Read the model definition and answer for the solid it produces. Units are mm, in the model's axes. A direction names the side the tool comes from. Give positions to 0.01 mm unless a question says otherwise; leave off trailing zeros. Write each loop counter-clockwise with the first axis right and the second up, starting at its lowest first coordinate (ties: lowest second). Pieces come first, ordered by that corner, then holes.
```python
from build123d import *

# Parameters (mm, degrees)
SKETCH1_W                      = 55.88
SKETCH1_H                      = 12.7
BOSS_EXTRUDE1_DEPTH            = 3.81
SKETCH2_W                      = 9.525
SKETCH2_H                      = 12.7
BOSS_EXTRUDE2_DEPTH            = 16.51
F_8_0_199_DIAMETER_HOLE1_D     = 5.0546
F_8_0_199_DIAMETER_HOLE1_DEPTH = 7.112
F_8_0_199_DIAMETER_HOLE1_TIP   = 1.518555042


with BuildPart() as part:
    # Sketch1 → Boss-Extrude1 (new body)
    with BuildSketch(Plane(origin=(0, 0, 0), x_dir=(1, 0, 0), z_dir=(0, 1, 0))):
        with Locations((-27.94, 6.35)):
            Rectangle(SKETCH1_W, SKETCH1_H)
    extrude(amount=BOSS_EXTRUDE1_DEPTH)

    # Sketch2 → Boss-Extrude2 (add)
    with BuildSketch(Plane(origin=(0, 3.81, 0), x_dir=(1, 0, 0), z_dir=(0, 1, 0))):
        with Locations((-51.1175, 6.35)):
            Rectangle(SKETCH2_W, SKETCH2_H)
        with Locations((-4.7625, 6.35)):
            Rectangle(SKETCH2_W, SKETCH2_H)
    extrude(amount=BOSS_EXTRUDE2_DEPTH)

    # #8 (0.199) Diameter Hole1
    with Locations(Plane(origin=(0, 20.32, 0), x_dir=(1, 0, 0), z_dir=(0, 1, 0))):
        with Locations((-50.8254, 6.505248616), (-5.0546, 6.505248616)):
            Hole(F_8_0_199_DIAMETER_HOLE1_D / 2, depth=F_8_0_199_DIAMETER_HOLE1_DEPTH)
            with Locations((0, 0, -(F_8_0_199_DIAMETER_HOLE1_DEPTH + F_8_0_199_DIAMETER_HOLE1_TIP / 2))):  # 118° drill point
                Cone(0, F_8_0_199_DIAMETER_HOLE1_D / 2, F_8_0_199_DIAMETER_HOLE1_TIP, mode=Mode.SUBTRACT)


solid = part.part
```
Item 1: Section C-C (z = -2.5) is taken. Write down the section's boundary in (x, y) (3 decimals), and give its area (3 significant figures).
Result set:
outline: (-55.88, 0) - (0, 0) - (0, 20.32) - (-9.525, 20.32) - (-9.525, 3.81) - (-46.355, 3.81) - (-46.355, 20.32) - (-55.88, 20.32) - close
area: 527 mm2
Item 2: Section A-A (y = 7) is taken. Write down the section's boundary in (x, z) (3 decimals).
Result set:
outline: (-55.88, -12.7) - (-46.355, -12.7) - (-46.355, 0) - (-55.88, 0) - close; (-9.525, -12.7) - (0, -12.7) - (0, 0) - (-9.525, 0) - close
Item 3: Which of the six approach directions +Z, -Z, +X, -X, +Y, -Y give full straight-line access (tool end or side, diameter ignored) to faces 1 (the flat face through (-53.3, 20.32, -5)), 2 (the cylindrical face through (-4.73, 16.71, -9.01)), 3 (the flat face through (-46.355, 12, -6))?
Result set:
face 1: +Z, -Z, +X, -X, +Y
face 2: +Y
face 3: +Z, -Z, +Y
Item 4: Section D-D (x = -11.5) is taken. Write down the section's boundary in (y, z).
Result set:
outline: (0, -12.7) - (3.81, -12.7) - (3.81, 0) - (0, 0) - close
Item 5: Determine the mould class of faces 4 (the flat face through (-55.88, 10, -6)), 5 (the flat face through (-2.7, 20.32, -5)), 6 (the flat face through (-9.525, 12, -6)), 7 (the conical face through (-4.819, 11.953, -6.875)) for opening direction X: pulls with the +X half, pulls with the -X half, needs draft (parallel to the pull), parting line crosses it, or undercut.
Result set:
face 4: pulls with the -X half
face 5: needs draft
face 6: undercut
face 7: undercut
Item 6: Section B-B (y = 16.25) is taken. Write down the section's boundary in (x, z) (3 decimals).
Result set:
outline: (-55.88, -12.7) - (-46.355, -12.7) - (-46.355, 0) - (-55.88, 0) - close; (-9.525, -12.7) - (0, -12.7) - (0, 0) - (-9.525, 0) - close; hole circle Ø5.055 at (-50.825, -6.505); hole circle Ø5.055 at (-5.055, -6.505)
Item 7: Find the intervals of material crossed by line 1 along X through (y, z) = (4.25, -2.25) (3 decimals); line 2 along X through (y, z) = (15.75, -7.25) (3 decimals); line 3 along X through (y, z) = (15, -8.75) (3 decimals), in increasing order.
Result set:
line 1: x = -55.88 to -46.355, -9.525 to 0
line 2: x = -55.88 to -53.24, -48.41 to -46.355, -9.525 to -7.47, -2.64 to 0
line 3: x = -55.88 to -51.987, -49.664 to -46.355, -9.525 to -6.216, -3.893 to 0
Item 8: This flat-tipped pin is pushed along its axis until it touches: pin 1 Ø1.5 at (x, z) = (-30.5, -9) entering from +Y. Where does it stop, or does it pass through?
Result set:
pin 1: stops at y = 3.81
